Source: CAD feature listing. Evaluate the final solid. Frame: model axes, mm. A direction names the side the tool comes from. Give positions to 0.01 mm unless a question says otherwise; leave off trailing zeros. Loops run counter-clockwise (first coordinate to the right, second up) from the corner with the lowest first, then second, coordinate; pieces in that order, holes last. Notation, with made-up numbers: M 40.5,-10 L 57.5,-10 A13 ccw 57.5,15 Z; hole C 26.25,4.5 d4. An arc over 180 degrees is marked long. Put each result on its own line as item: value.
from build123d import *

# Parameters (mm, degrees)
SKETCH1_W           = 20
SKETCH1_H           = 20
BOSS_EXTRUDE1_DEPTH = 101.6
CUT_EXTRUDE1_DEPTH  = 203.2
SKETCH3_R           = 2.1
CUT_EXTRUDE2_DEPTH  = 13
CUT_EXTRUDE3_START  = -13
SKETCH4_R           = 2.1
CUT_EXTRUDE3_DEPTH  = 13


with BuildPart() as part:
    # Sketch1 → Boss-Extrude1 (new, symmetric)
    with BuildSketch(Plane(origin=(0, 0, 0), x_dir=(1, 0, 0), z_dir=(0, 1, 0))):
        Rectangle(SKETCH1_W, SKETCH1_H)
    extrude(amount=BOSS_EXTRUDE1_DEPTH, both=True)

    # Sketch2 → Cut-Extrude1 (cut)
    with BuildSketch(Plane(origin=(0, 101.6, 0), x_dir=(1, 0, 0), z_dir=(0, 1, 0))):
        Polygon((-10, -3), (-10, 3), (-8, 3), (-8, 6), (-4.000000001, 3), (-4.000000001, -3), (-8, -6), (-8, -3), align=None)
        Polygon((3, 4.000000001), (6, 8), (3, 8), (3, 10), (-3, 10), (-3, 8), (-6, 8), (-3, 4.000000001), align=None)
        Polygon((4.000000001, -3), (8, -6), (8, -3), (10, -3), (10, 3), (8, 3), (8, 6), (4.000000001, 3), align=None)
        Polygon((-3, -4.000000001), (-6, -8), (-3, -8), (-3, -10), (3, -10), (3, -8), (6, -8), (3, -4.000000001), align=None)
    extrude(amount=-CUT_EXTRUDE1_DEPTH, mode=Mode.SUBTRACT)

    # Sketch3 → Cut-Extrude2 (cut)
    with BuildSketch(Plane(origin=(0, 101.6, 0), x_dir=(1, 0, 0), z_dir=(0, 1, 0))):
        with Locations(Location((0, 0, 0), (0, 0, 270))):
            Circle(SKETCH3_R)
    extrude(amount=-CUT_EXTRUDE2_DEPTH, mode=Mode.SUBTRACT)

    # Sketch4 → Cut-Extrude3 (cut)
    with BuildSketch(Plane.XZ.offset(101.6).offset(CUT_EXTRUDE3_START)):
        with Locations(Location((0, 0, 0), (0, 0, 90))):
            Circle(SKETCH4_R)
    extrude(amount=CUT_EXTRUDE3_DEPTH, mode=Mode.SUBTRACT)


solid = part.part
1. Access query for faces 4 (the flat face through (-4, 1, 0)), 5 (the flat face through (0, -88.6, 0)), 6 (the cylindrical face through (0.631, 95.191, 2.003)), 7 (the flat face through (-10, 1, 7)), 8 (the flat face through (0, 1, 4)). Directions: +Z, -Z, +X, -X, +Y, -Y. A direction counts if a zero-diameter tool reaches every point of the face in a straight line with its end or side. Return the directions, or none.
Found:
face 4: -X, +Y, -Y
face 5: -Y
face 6: +Y
face 7: +Z, -Z, -X, +Y, -Y
face 8: +Z, +Y, -Y
2. Contact query for flat-ended pins moving along their axis: P1, Ø1.3, axis at x = -0.5, z = 1, coming from the -Y side; P2, Ø1.3, axis at x = 1, z = 1, coming from the +Y side; P3, Ø1.8, axis at x = 1, y = -25.5, coming from the -Z side. Output: stop coordinate, or through.
Found:
P1: y = -88.6
P2: y = 88.6
P3: z = -4
3. Section query B-B (z = 0). Output: boundary loops of the cut face in (x, y).
Found:
outline: M -4,-101.6 L -2.1,-101.6 L -2.1,-88.6 L 2.1,-88.6 L 2.1,-101.6 L 4,-101.6 L 4,101.6 L 2.1,101.6 L 2.1,88.6 L -2.1,88.6 L -2.1,101.6 L -4,101.6 Z
4. Draft query along Z for faces 1 (the flat face through (4.5, 1.4, -6)), 2 (the flat face through (0, 1, -4)), 3 (the flat face through (-7, 1, 10)). Return one class per face: pulls with the +Z half, pulls with the -Z half, needs draft (parallel to the pull), parting line crosses it, or undercut.
Found:
face 1: undercut
face 2: pulls with the -Z half
face 3: pulls with the +Z half
5. Section query A-A (x = 0). Output: boundary loops of the cut face in (y, z), plus the area to 3 significant figures.
Found:
outline: M -101.6,-4 L 101.6,-4 L 101.6,-2.1 L 88.6,-2.1 L 88.6,2.1 L 101.6,2.1 L 101.6,4 L -101.6,4 L -101.6,2.1 L -88.6,2.1 L -88.6,-2.1 L -101.6,-2.1 Z
area: 1,520 mm^2
6. Material intervals for line 1 (Z direction, x = -8.75, y = 31.5); line 2 (Z direction, x = -5.5, y = -65) (3 decimals); line 3 (Z direction, x = -3.25, y = -72), sorted ascending. Write a range as from..to.
Found:
line 1: -10..-3, 3..10
line 2: -10..-8, -7.333..-4.125, 4.125..7.333, 8..10
line 3: -10..-8, -4.33..4.33, 8..10
